For this review, use the dimensioned drawing (mm, ordinates from the lowest corner) and the shaded views. A direction names the side the tool comes from. Give positions to 0.01 mm unless a question says otherwise; leave off trailing zeros. Write each loop counter-clockwise with the first axis right and the second up, starting at its lowest first coordinate (ties: lowest second). Pieces come first, ordered by that corner, then holes.
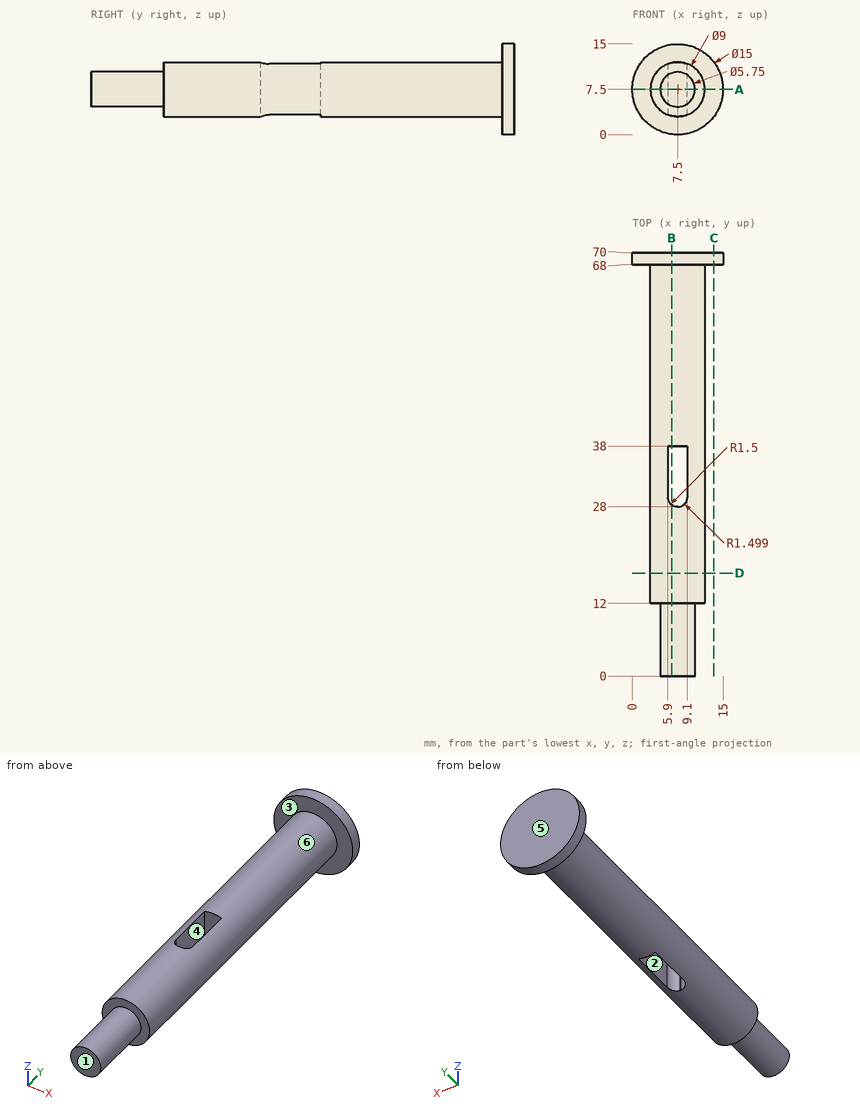
(1) We need section B-B (x = 6.5). Write out the cut boundary in (y, z).
(2) We need section D-D (y = 17). Write out the cut boundary in (x, z).
(3) We need section A-A (z = 7.5). Write out the cut boundary in (x, y) (3 decimals), and give its area (3 significant figures).
(4) Clearance check with flat-ended pins moving along their axes: pin 1 Ø6.5 at (y, z) = (35.5, 7.5) entering from +X; pin 2 Ø2 at (x, y) = (8.5, 43.5) entering from -Z; pin 3 Ø3 at (y, z) = (37, 2) entering from -X. State where each tip first meets the part, or that it passes through.
(5) We need section C-C (x = 13.5). Write out the cut boundary in (y, z).
(6) The part is to be moulded in two halves that separate along X. For the marked faces 4, 5 and 6, say which applies: +X half, -X half, draft (parallel to the pull), parting line (faces both ways), or undercut.
(7) For L1, parallel to Y at x = 11.75, z = 5.5; L2, parallel to X at y = 31, z = 8.25; L3, parallel to Y at x = 8.25, z = 6.75, list the stretches that pass through material, from the lowest coordinate up.
(8) Tool access review of the marked faces 1, 2 and 3: name each direction out of +Z, -Z, +X, -X, +Y, -Y from which nothing blocks a thin tool from reaching the whole face with its end or side.
The answers:
1. outline: (0, 4.8) - (12, 4.8) - (12, 3.11) - (28.3, 3.11) - (28.3, 11.89) - (12, 11.89) - (12, 10.2) - (0, 10.2) - close; (38, 3.11) - (68, 3.11) - (68, 0.07) - (70, 0.07) - (70, 14.93) - (68, 14.93) - (68, 11.89) - (38, 11.89) - close
2. outline: circle Ø9 at (7.5, 7.5)
3. outline: (0, 68) - (3, 68) - (3, 12) - (4.625, 12) - (4.625, 0) - (10.375, 0) - (10.375, 12) - (12, 12) - (12, 68) - (15, 68) - (15, 70) - (0, 70) - close; hole (5.9, 29.5) arc R1.5 ccw to (7.4, 28) - (7.601, 28) arc R1.499 ccw to (9.1, 29.499) - (9.1, 38) - (5.9, 38) - close
3. area: 572 mm2
4. pin 1: stops at x = 12
4. pin 2: stops at z = 3
4. pin 3: stops at x = 5.44
5. outline: (68, 3) - (70, 3) - (70, 12) - (68, 12) - close
6. face 4: undercut
6. face 5: draft
6. face 6: parting line
7. L1: y = 68 to 70
7. L2: x = 3.06 to 5.9, 9.1 to 11.94
7. L3: y = 0 to 28.15, 38 to 70
8. face 1: +Z, -Z, +X, -X, -Y
8. face 2: +Z, -Z
8. face 3: -Y
